The listing builds one solid part. Answer for the finished solid, in the listing's coordinates (mm). Face numbers are marked on the shaded views. Coordinates: 2 decimals unless noted, no trailing zeros. Write each loop counter-clockwise with the first axis right and the second up, starting at its lowest first coordinate (ties: lowest second). Pieces come first, ordered by that corner, then holes. Notation, with made-up numbers: M -34.5,89.5 L 11.5,89.5 A25 cw 11.5,103.5 Z; hole C -13,-23.5 d2. An arc over 180 degrees is marked long. Put each result on its own line as item: value. Start each with the question number.
```python
from build123d import *

# Parameters (mm, degrees)
SKETCH_1_W               = 10
SKETCH_1_H               = 11
CHAMFER_1_SIZE           = 2
SKETCH_2_R               = 6
CUT_EXTRUDE_1_DEPTH      = 19.493242009
CUT_EXTRUDE_2_DEPTH      = 19.493242009
CUT_EXTRUDE_2_DEPTH_BACK = 19.493242009
SKETCH_3_R               = 2


with BuildPart() as part:
    # 草图1 → 旋转1 (revolve)
    with BuildSketch(Plane.XY, mode=Mode.PRIVATE) as revolve_1_sk:
        with Locations((-5, 5.5)):
            Rectangle(SKETCH_1_W, SKETCH_1_H)
    revolve(revolve_1_sk.sketch.rotate(Axis((0, 0, 0), (-1, 0, 0)), 90), axis=Axis((0, 0, 0), (-1, 0, 0)))

    # 倒角1
    chamfer_1_edges = [part.edges().sort_by_distance(p)[0] for p in [
        (-10, 0, 11),
    ]]
    chamfer(chamfer_1_edges, length=CHAMFER_1_SIZE)

    # 草图2 → 切除-拉伸1 (cut, through all)
    with BuildSketch(Plane.ZY.offset(10)):
        Circle(SKETCH_2_R)
    extrude(amount=-CUT_EXTRUDE_1_DEPTH, mode=Mode.SUBTRACT)

    # 草图3 → 切除-拉伸2 (cut, two sides: drawn at the far end of the back side and taken through both)
    with BuildSketch(Plane(origin=(0, 0, 0), x_dir=(1, 0, 0), z_dir=(0, 1, 0)).offset(-CUT_EXTRUDE_2_DEPTH_BACK)):
        with Locations(Location((-5, 0, 0), (0, 0, 270))):
            Circle(SKETCH_3_R)
    extrude(amount=CUT_EXTRUDE_2_DEPTH + CUT_EXTRUDE_2_DEPTH_BACK, mode=Mode.SUBTRACT)


solid = part.part
```
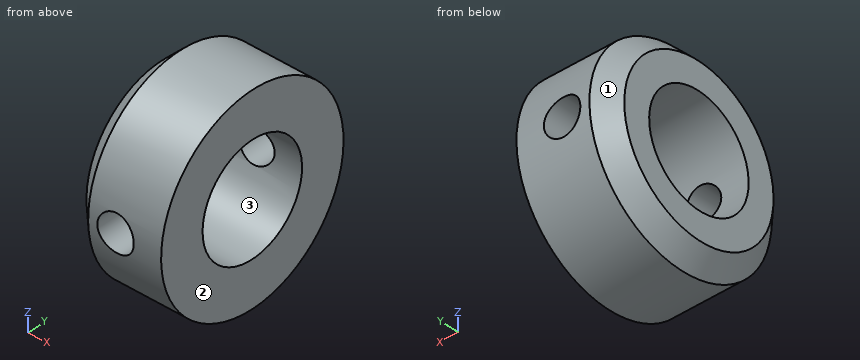
1) Given pin 1 Ø11 at (y, z) = (0, 0) entering from +X; pin 2 Ø1 at (x, z) = (-7, 1.5) entering from +Y, each flat-ended and moving along its own axis, determine where each tip first touches the part or whether it passes through.
2) A cutting plane is placed at B-B on y = 0. Write down the section's boundary in (x, z), then the cut area to 3 significant figures.
3) A cutting plane is placed at C-C on x = -5. Write down the section's boundary in (y, z).
4) Determine the mould class of the marked faces 1, 2 and 3 for opening direction Y: +Y half, -Y half, draft (parallel to the pull), parting line (faces both ways), or undercut.
5) A cutting plane is placed at A-A on z = 0. Write down the section's boundary in (x, y), then the cut area to 3 significant figures.
6) A cutting plane is placed at D-D on x = -2.25. Write down the section's boundary in (y, z).
7) Straight lines are drawn through the part: probe 1 along X at (y, z) = (8.6, 0); probe 2 along Y at (x, z) = (-4.75, 2.25); probe 3 along Z at (x, y) = (-5, 9.15). For each, find the intervals that lie inside material, in ascending order.
Answers follow:
1. pin 1: passes through
1. pin 2: stops at y = 10.95
2. outline: M -10,-9 L -8,-11 L 0,-11 L 0,-6 L -10,-6 Z; M -10,6 L 0,6 L 0,11 L -8,11 L -10,9 Z
2. area: 96.0 mm²
3. outline: M -10.82,-2 A11 ccw 10.82,-2 L 5.66,-2 A6 cw -5.66,-2 Z; M -10.82,2 L -5.66,2 A6 cw 5.66,2 L 10.82,2 A11 ccw Z
4. face 1: parting line
4. face 2: draft
4. face 3: undercut
5. outline: M -10,-9 L -8,-11 L -7,-11 L -7,-6 L -10,-6 Z; M -10,6 L -7,6 L -7,11 L -8,11 L -10,9 Z; M -3,-11 L 0,-11 L 0,-6 L -3,-6 Z; M -3,6 L 0,6 L 0,11 L -3,11 Z
5. area: 56.0 mm²
6. outline: C 0,0 d22; hole C 0,0 d12
7. probe 1: x = -10 to -7, -3 to 0
7. probe 2: y = -10.77 to -5.56, 5.56 to 10.77
7. probe 3: z = -6.11 to -2, 2 to 6.11
